```python
from build123d import *

# Parameters (mm, degrees)
SKETCH_1_W          = 27.94
SKETCH_1_H          = 3
EXTRUDE_2_DEPTH     = 6
SKETCH_2_W          = 3
SKETCH_2_H          = 1.5
CUT_EXTRUDE_1_DEPTH = 6
CHAMFER_1_SIZE      = 0.5
CHAMFER_2_SIZE      = 0.5
SKETCH_3_W          = 12
SKETCH_3_H          = 2
CUT_EXTRUDE_2_DEPTH = 16.49712554


with BuildPart() as part:
    # Эскиз1 → Бобышка-Вытянуть2 (new body)
    with BuildSketch(Plane.XY):
        Rectangle(SKETCH_1_W, SKETCH_1_H)
    extrude(amount=EXTRUDE_2_DEPTH)

    # Эскиз2 → Вырез-Вытянуть1 (cut)
    with BuildSketch(Plane(origin=(0, 1.5, 0), x_dir=(1, 0, 0), z_dir=(0, 1, 0))):
        with Locations((-9.97, -1.75)):
            Rectangle(SKETCH_2_W, SKETCH_2_H)
        with Locations((-9.97, -4.25)):
            Rectangle(SKETCH_2_W, SKETCH_2_H)
        with Locations((9.97, -4.25)):
            Rectangle(SKETCH_2_W, SKETCH_2_H)
        with Locations((9.97, -1.75)):
            Rectangle(SKETCH_2_W, SKETCH_2_H)
    extrude(amount=-CUT_EXTRUDE_1_DEPTH, mode=Mode.SUBTRACT)

    # Фаска1
    chamfer_1_edges = [part.edges().sort_by_distance(p)[0] for p in [
        (0, 1.5, 0),
        (0, 1.5, 6),
        (-13.97, 1.5, 3),
        (13.97, 1.5, 3),
    ]]
    chamfer(chamfer_1_edges, length=CHAMFER_1_SIZE)

    # Фаска2
    chamfer_2_edges = [part.edges().sort_by_distance(p)[0] for p in [
        (0, -1.5, 6),
        (0, -1.5, 0),
        (13.97, -1.5, 3),
        (-13.97, -1.5, 3),
    ]]
    chamfer(chamfer_2_edges, length=CHAMFER_2_SIZE)

    # Эскиз3 → Вырез-Вытянуть2 (cut, through all)
    with BuildSketch(Plane(origin=(0, 1.5, 0), x_dir=(1, 0, 0), z_dir=(0, 1, 0))):
        with Locations((0, -3)):
            Rectangle(SKETCH_3_W, SKETCH_3_H)
    extrude(amount=-CUT_EXTRUDE_2_DEPTH, mode=Mode.SUBTRACT)


solid = part.part
```
Can you work these out from the model? Positions are in its coordinate system, mm. A direction names the side the tool comes from. Give positions to 0.01 mm unless a question says otherwise; leave off trailing zeros. Order: outer loops, then holes, each group sorted by start corner. A loop starts at its lowest first (then second) coordinate and runs counter-clockwise, first axis right, second up. Notation, with made-up numbers: (-26.5, -31) - (28.5, -31) arc R24 ccw to (28.5, 8) - close; hole circle Ø10 at (23, 68). An arc over 180 degrees is marked (long way). Use a Markdown table: item, result. Add a question column.
Q1. If we section it at D-D on y = 0.55: Write out the boundary of the cut face in (x, z).
Q2. If we section it at A-A on z = 2.75: Write out the boundary of the cut face in (x, y), plus the area to 3 significant figures.
Q3. If we section it at C-C on z = 1.6: Write out the boundary of the cut face in (x, y), plus the area to 3 significant figures.
Q4. Please list where these lines run through material, in increasing order: line 1 along X through (y, z) = (-0.4, 1.7); line 2 along X through (y, z) = (-0.45, 3.8); line 3 along Z through (x, y) = (-1.75, 0.35).
Q5. On a 3-axis mill with a long thin cutter (end or side, diameter ignored), from which of +Z, -Z, +X, -X, +Y, -Y can I reach the whole of each face in a straight line? I mean faces 4 (the flat face through (0, 0, 0)), 5 (the flat face through (10, 0, 5)). Say none if no direction works.
Q6. If we mould it in two halves opening along X, with no side actions, what happens to faces 1 (the flat face through (0, 0, 6)), 2 (the flat face through (13.97, 0, 3)), 3 (the flat face through (-10, 0, 3.5))? For each: released by +X, released by -X, zero draft, split by the parting line, or undercut.
Q7. If we section it at B-B on x = 3: Write out the boundary of the cut face in (y, z).
Answers follow:
| question | item | result |
|---|---|---|
| 1 | outline | (-13.97, 0) - (13.97, 0) - (13.97, 6) - (-13.97, 6) - close; hole (-11.47, 1) - (-8.47, 1) - (-8.47, 2.5) - (-11.47, 2.5) - close; hole (-11.47, 3.5) - (-8.47, 3.5) - (-8.47, 5) - (-11.47, 5) - close; hole (-6, 2) - (6, 2) - (6, 4) - (-6, 4) - close; hole (8.47, 1) - (11.47, 1) - (11.47, 2.5) - (8.47, 2.5) - close; hole (8.47, 3.5) - (11.47, 3.5) - (11.47, 5) - (8.47, 5) - close |
| 2 | outline | (-13.97, -1) - (-13.47, -1.5) - (-6, -1.5) - (-6, 1.5) - (-13.47, 1.5) - (-13.97, 1) - close; (6, -1.5) - (13.47, -1.5) - (13.97, -1) - (13.97, 1) - (13.47, 1.5) - (6, 1.5) - close |
| 2 | area | 47.3 mm^2 |
| 3 | outline | (-13.97, -1) - (-13.47, -1.5) - (-11.47, -1.5) - (-11.47, 1.5) - (-13.47, 1.5) - (-13.97, 1) - close; (-8.47, -1.5) - (8.47, -1.5) - (8.47, 1.5) - (-8.47, 1.5) - close; (11.47, -1.5) - (13.47, -1.5) - (13.97, -1) - (13.97, 1) - (13.47, 1.5) - (11.47, 1.5) - close |
| 3 | area | 65.3 mm^2 |
| 4 | line 1 | x = -13.97 to -11.47, -8.47 to 8.47, 11.47 to 13.97 |
| 4 | line 2 | x = -13.97 to -11.47, -8.47 to -6, 6 to 8.47, 11.47 to 13.97 |
| 4 | line 3 | z = 0 to 2, 4 to 6 |
| 5 | face 4 | -Z, +X, -X, +Y, -Y |
| 5 | face 5 | +Y, -Y |
| 6 | face 1 | zero draft |
| 6 | face 2 | released by +X |
| 6 | face 3 | undercut |
| 7 | outline | (-1.5, 0.5) - (-1, 0) - (1, 0) - (1.5, 0.5) - (1.5, 2) - (-1.5, 2) - close; (-1.5, 4) - (1.5, 4) - (1.5, 5.5) - (1, 6) - (-1, 6) - (-1.5, 5.5) - close |
